Check sheet for the modelled part. Datum: model origin and axes. Units: mm. A direction names the side the tool comes from. Round coordinates to 2 decimals unless told otherwise and drop trailing zeros. Write each loop counter-clockwise with the first axis right and the second up, starting at its lowest first coordinate (ties: lowest second). Pieces come first, ordered by that corner, then holes.
Item 1: Cross-section at C-C on z = 22.5. Enter the section's corners in (x, y).
Item 2: Go/stop test with flat-tipped pins: pin 1 Ø0.9 at (x, z) = (0.5, 48.5) entering from -Y; pin 2 Ø1.5 at (y, z) = (-2, -2) entering from -X; pin 3 Ø2 at (y, z) = (2.5, 49) entering from +X. Record where each tip stops, or that it passes through.
Item 3: Cross-section at B-B on x = -9. Enter the section's corners in (y, z).
Item 4: Material ranges on line 1 (Y direction, x = -28.8, z = -43); line 2 (X direction, y = 0.75, z = 6.5); line 3 (Z direction, x = -10, y = 0.75), recorded low to high.
Item 5: Tool access check on faces 1 (the flat face through (0, 2.885, 49)), 2 (the flat face through (-25, 1, -43)), 3 (the cylindrical face through (28, 3, -49)). Record the directions out of +Z, -Z, +X, -X, +Y, -Y that give a thin tool (end or side, any length) a straight path to the whole face; none if there is none.
Item 6: Release check for a two-part mould opening along X. For faces 4 (the flat face through (-11.5, 2, 49)), 5 (the cylindrical face through (29, 3, 48)), 6 (the flat face through (-30, 3, 1)) record: +X half, -X half, draft (parallel to the pull), parting line (faces both ways), or undercut.
Item 7: Cross-section at A-A on z = -43. Enter the section's corners in (x, y).
from build123d import *

# Parameters (mm, degrees)
BOSS_EXTRUDE1_DEPTH = 4
FILLET1_R           = 5
SKETCH4_W           = 23
SKETCH4_H           = 2
CUT_EXTRUDE1_DEPTH  = 3
SKETCH5_R           = 1.5
CUT_EXTRUDE2_DEPTH  = 5
CUT_EXTRUDE3_DEPTH  = 1


with BuildPart() as part:
    # Sketch1 → Boss-Extrude1 (new, symmetric)
    with BuildSketch(Plane(origin=(0, 0, 0), x_dir=(1, 0, 0), z_dir=(0, 1, 0))):
        with BuildLine():
            Line((25, -50), (-25, -50))
            ThreePointArc((-25, -50), (-28.535533906, -48.535533906), (-30, -45))
            Line((-30, -45), (-30, 45))
            ThreePointArc((-30, 45), (-28.535533906, 48.535533906), (-25, 50))
            Line((-25, 50), (25, 50))
            ThreePointArc((25, 50), (28.535533906, 48.535533906), (30, 45))
            Line((30, 45), (30, -45))
            ThreePointArc((30, -45), (28.535533906, -48.535533906), (25, -50))
        make_face()
    extrude(amount=BOSS_EXTRUDE1_DEPTH, both=True)

    # Fillet1
    fillet1_edges = [part.edges().sort_by_distance(p)[0] for p in [
        (0, -4, -50),
        (28.535533906, -4, -48.535533906),
        (30, -4, 0),
        (28.535533906, -4, 48.535533906),
        (0, -4, 50),
        (-28.535533906, -4, 48.535533906),
        (-30, -4, 0),
        (-28.535533906, -4, -48.535533906),
    ]]
    fillet(fillet1_edges, radius=FILLET1_R)

    # Sketch4 → Cut-Extrude1 (cut)
    with BuildSketch(Plane.XY.offset(50)):
        with Locations((0, 1.884621544)):
            Rectangle(SKETCH4_W, SKETCH4_H)
    extrude(amount=-CUT_EXTRUDE1_DEPTH, mode=Mode.SUBTRACT)

    # Sketch5 → Cut-Extrude2 (cut)
    with BuildSketch(Plane.ZY.offset(30)):
        with Locations((-43, 1)):
            Circle(SKETCH5_R)
    extrude(amount=-CUT_EXTRUDE2_DEPTH, mode=Mode.SUBTRACT)

    # Sketch6 → Cut-Extrude3 (cut)
    with BuildSketch(Plane.ZY.offset(30)):
        with BuildLine():
            Line((34.15, 2.5), (43.15, 2.5))
            ThreePointArc((43.15, 2.5), (44.65, 1), (43.15, -0.5))
            Line((43.15, -0.5), (34.15, -0.5))
            ThreePointArc((34.15, -0.5), (32.65, 1), (34.15, 2.5))
        make_face()
    extrude(amount=-CUT_EXTRUDE3_DEPTH, mode=Mode.SUBTRACT)


solid = part.part
Response values:
1. outline: (-30, 1) arc R5 ccw to (-25, -4) - (25, -4) arc R5 ccw to (30, 1) - (30, 4) - (-30, 4) - close
2. pin 1: stops at y = -2.96
2. pin 2: stops at x = -29.47
2. pin 3: stops at x = 29
3. outline: (-4, -45) arc R5 ccw to (1, -50) - (4, -50) - (4, 50) - (2.88, 50) - (2.88, 47) - (0.88, 47) - (0.88, 50) arc R5 ccw to (-4, 45) - close
4. line 1: y = -2.25 to -0.5, 2.5 to 4
4. line 2: x = -29.99 to 29.99
4. line 3: z = -49.99 to 49.99
5. face 1: +Z
5. face 2: -X
5. face 3: -Z, +X, +Y, -Y
6. face 4: undercut
6. face 5: +X half
6. face 6: -X half
7. outline: (-30, 2.5) - (-25, 2.5) - (-25, -0.5) - (-29.77, -0.5) arc R5 ccw to (-25, -4) - (25, -4) arc R5 ccw to (30, 1) - (30, 4) - (-30, 4) - close
